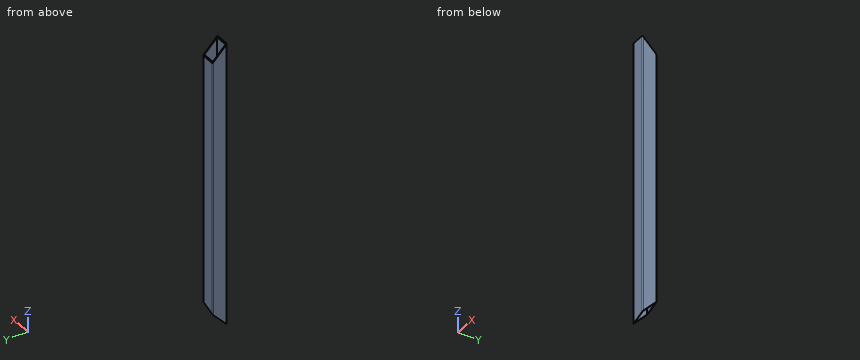
from build123d import *

# Parameters (mm, degrees)
F0_W          = 44.45
F0_H          = 44.45
F1_DEPTH      = 1003.3
F3_DEPTH      = 50.801
F5_DEPTH      = 50.801
F7_W          = 181.430888
F7_H          = 203.2
F8_DEPTH      = 50.8
F8_DEPTH_BACK = 6.35


with BuildPart() as f1:
    # F0 (on Top) → F1 (new body)
    with BuildSketch(Plane.XY):
        with BuildLine():
            ThreePointArc((25.4, 22.225), (24.470064, 24.470064), (22.225, 25.4))
            Line((22.225, 25.4), (-22.225, 25.4))
            ThreePointArc((-22.225, 25.4), (-24.470064, 24.470064), (-25.4, 22.225))
            Line((-25.4, 22.225), (-25.4, -22.225))
            ThreePointArc((-25.4, -22.225), (-24.470064, -24.470064), (-22.225, -25.4))
            Line((-22.225, -25.4), (22.225, -25.4))
            ThreePointArc((22.225, -25.4), (24.470064, -24.470064), (25.4, -22.225))
            Line((25.4, -22.225), (25.4, 22.225))
        make_face()
        Rectangle(F0_W, F0_H, mode=Mode.SUBTRACT)
    extrude(amount=F1_DEPTH)

    # F2 (on face) → F3 (cut, through all)
    with BuildSketch(Plane.YZ.offset(25.4)):
        Polygon((25.4, 1003.3), (-25.4, 1003.3), (25.4, 952.5), align=None)
    extrude(amount=-F3_DEPTH, mode=Mode.SUBTRACT)

    # F4 (on face) → F5 (cut, through all)
    with BuildSketch(Plane.XZ.offset(25.4)):
        Polygon((-25.4, 0), (25.4, 0), (25.4, 18.489688), align=None)
    extrude(amount=-F5_DEPTH, mode=Mode.SUBTRACT)

    # F7 (on face) → F8 (cut, two sides)
    with BuildSketch(Plane(origin=(-5.286317, -15.456156, 14.524036), x_dir=(-0.970315, 0.176242, -0.165613), z_dir=(0.241845, 0.707107, -0.664463))) as f8_sk:
        with Locations((-6.846333, -13.58029)):
            Rectangle(F7_W, F7_H)
    extrude(amount=F8_DEPTH, mode=Mode.SUBTRACT)
    extrude(f8_sk.sketch, amount=-F8_DEPTH_BACK, mode=Mode.SUBTRACT)


solid = f1.part
Verification items for the finished model (mm, model axes). Give positions to 0.01 mm unless a question says otherwise; leave off trailing zeros. Write each loop counter-clockwise with the first axis right and the second up, starting at its lowest first coordinate (ties: lowest second). Pieces come first, ordered by that corner, then holes. Notation, with made-up numbers: (4, -1.75) - (58, -1.75) arc R21 cw to (58, 7.25) - close; hole circle Ø3 at (-13.5, -22.5). An arc over 180 degrees is marked (long way). Answer as CSV lines item,"result". Start each with the question number.
1. Sectioned sample at C-C (x = -4). Record the boundary of the cut face in (y, z) (3 decimals), then the cut area to 3 significant figures.
2. Sectioned sample at B-B (z = 606). Record the boundary of the cut face in (x, y) (3 decimals).
3. Thickness scan on line 1 (X direction, y = 11.5, z = 225.5) (3 decimals); line 2 (Z direction, x = 20, y = 22.5). Record the ranges inside material, lowest first.
4. Sectioned sample at A-A (y = -3). Record the boundary of the cut face in (x, z) (1 decimal), then the cut area to 3 significant figures.
Derived:
1,outline,"(-25.4, 13.967) - (-22.225, 17.346) - (-22.225, 1000.125) - (-25.4, 1003.3) - close; (22.225, 64.648) - (25.4, 68.027) - (25.4, 952.5) - (22.225, 955.675) - close"
1,area,"5,950 mm²"
2,outline,"(-25.4, -22.225) arc R3.175 ccw to (-22.225, -25.4) - (22.225, -25.4) arc R3.175 ccw to (25.4, -22.225) - (25.4, 22.225) arc R3.175 ccw to (22.225, 25.4) - (-22.225, 25.4) arc R3.175 ccw to (-25.4, 22.225) - close; hole (-22.225, -22.225) - (22.225, -22.225) - (22.225, 22.225) - (-22.225, 22.225) - close"
3,line 1,"-25.4 to -22.225, 22.225 to 25.4"
3,line 2,"73.68 to 955.4"
4,outline,"(-25.4, 30) - (-22.2, 31.2) - (-22.2, 980.9) - (-25.4, 980.9) - close; (22.2, 47.3) - (25.4, 48.5) - (25.4, 980.9) - (22.2, 980.9) - close"
4,area,"5,980 mm²"
